Autodesk Inventor part; units mm, degrees
ref_plane "YZ Plane" through (0, 0, 0) normal (1, 0, 0) x (0, 1, 0)
ref_plane "XZ Plane" through (0, 0, 0) normal (0, 1, 0) x (-1, 0, 0)
ref_plane "XY Plane" through (0, 0, 0) normal (0, 0, 1) x (1, 0, 0)
sketch "Sketch1" plane through (0, 0, 0) normal (0, 1, 0) x (-1, 0, 0)
  line L0 (6.1765, 12) -> (-98.8235, 12)
  line L1 (-98.8235, 12) -> (-98.8235, -102)
  line L2 (-6.8235, 12) -> (-6.8235, 18)
  line L3 (-6.8235, 18) -> (6.1765, 18)
  line L4 (6.1765, 18) -> (6.1765, 12)
  line L5 (-98.8235, 12) -> (-98.8235, 18)
  line L6 (-98.8235, 18) -> (-85.8235, 18)
  line L7 (-85.8235, 18) -> (-85.8235, 12)
  line L8 (-98.8235, -102) -> (-85.8235, -87.8857)
  line L9 (-6.8235, -2.1143) -> (6.1765, 12)
  line L10 (-98.8235, -102) -> (-80.8235, -102)
  line L11 (6.1765, 12) -> (-80.8235, -102)
  point P0 (0, 0)
  point P1 (-96.8235, 18)
  point P2 (-96.8235, 18)
  dimension "d0" = 114
  dimension "d1" = 105
  dimension "d2" = 13
  dimension "d3" = 6
  dimension "d4" = 13
  dimension "d5" = 6
  dimension "d6" = 18
extrude "Extrusion1" add sketch "Sketch1" along normal blind 2
sketch "Sketch2" plane through (0, 2, 0) normal (0, 1, 0) x (1, 0, 0)
  line L0 (98.8235, 102) -> (80.8235, 102)
  line L1 (95.8235, 102) -> (87.8235, 102)
  line L2 (87.8235, 102) -> (87.8235, 82)
  line L3 (87.8235, 82) -> (95.8235, 82)
  line L4 (95.8235, 82) -> (95.8235, 102)
  line L5 (98.8235, -18) -> (98.8235, 102)
  point P0 (0, 0)
  dimension "d9" = 20
  dimension "d10" = 8
  dimension "d11" = 3
extrude "Extrusion2" add sketch "Sketch2" along normal blind 3
fillet "Fillet1" radius 4 2 edges at (87.8235, 5, -92) (95.8235, 5, -92)
sketch "Sketch3" plane through (0, 0, 0) normal (0, -1, 0) x (1, 0, 0)
  line L0 (87.8235, -102) -> (80.8235, -102)
  line L1 (87.8235, -102) -> (95.8235, -102)
  line L2 (95.8235, -102) -> (95.8235, -82)
  line L3 (95.8235, -82) -> (87.8235, -82)
  line L4 (87.8235, -82) -> (87.8235, -102)
  line L5 (98.8235, 18) -> (98.8235, -102)
  point P0 (0, 0)
  dimension "d16" = 20
  dimension "d17" = 8
  dimension "d18" = 3
extrude "Extrusion3" add sketch "Sketch3" along normal blind 3
fillet "Fillet3" radius 4 2 edges at (87.8235, -3, -92) (95.8235, -3, -92)
sketch "Sketch4" plane through (80.8235, 0, -102) normal (0, 0, -1) x (-1, 0, 0)
  arc A0 (-15, 0) -> (-11.127, -3) centre (-11.127, 1) ccw
  line L0 (-11.127, 4.8105) -> (-11.127, -3)
  circle A1 centre (-11.127, 1) radius 2.5
  point P0 (80.8235, 0)
  dimension "d25" = 5
extrude "Extrusion4" cut sketch "Sketch4" against normal blind 5
sketch "Sketch5" plane through (0, 2, 0) normal (0, 1, 0) x (1, 0, 0)
  line L0 (85.8235, -12) -> (85.8235, -18)
  line L1 (85.8235, -12) -> (98.8235, -12)
  line L2 (98.8235, -18) -> (98.8235, 102)
  circle A0 centre (92.3235, -12) radius 2.5
  point P0 (0, 0)
  dimension "d26" = 5
extrude "Extrusion5" cut sketch "Sketch5" against normal blind 2
sketch "Sketch6" plane through (0, 2, 0) normal (0, 1, 0) x (1, 0, 0)
  line L0 (-6.1765, -12) -> (-6.1765, -18)
  line L1 (6.8235, -18) -> (6.8235, -12)
  line L2 (-6.1765, -12) -> (6.8235, -12)
  circle A0 centre (0.3235, -12) radius 2.5
  point P0 (0, 0)
  dimension "d29" = 5
  dimension "d32" = 6.5
  dimension "d33" = 6
extrude "Extrusion6" cut sketch "Sketch6" against normal blind 2
equation "\"d23\" = d22"
properties part number "Triangle"
Can you work these out from the model? Positions are in its coordinate system, mm. A direction names the side the tool comes from. Give positions to 0.01 mm unless a question says otherwise; leave off trailing zeros. Loops run counter-clockwise (first coordinate to the right, second up) from the corner with the lowest first, then second, coordinate; pieces in that order, holes last. Notation, with made-up numbers: (23, 52) -> (76, 52) arc R31 cw to (76, 90) -> close; hole circle Ø6 at (-29.75, 82). An arc over 180 degrees is marked (long way). Write item = value, one per line.
1) Suppose I cut it at B-B on x = 52. Write out the boundary of the cut face in (y, z).
Check result:
outline = (0, -64.23) -> (2, -64.23) -> (2, 12) -> (0, 12) -> close
2) Thinking about a two-plate mould opening in X: for faces 1 (the flat face through (92, 1, -97)), 2 (the cylindrical face through (94.43, 4.14, -91.86)), 3 (the flat face through (92, -1, -82)), which applies, released by +X, released by -X, zero draft, split by the parting line, or undercut?
Check result:
face_1 = undercut
face_2 = released by +X
face_3 = zero draft
3) Suppose I cut it at A-A on z = -89. Write out the boundary of the cut face in (x, y).
Check result:
outline = (70.9, 0) -> (87.82, 0) arc R4 ccw to (91.7, -3) -> (91.95, -3) arc R4 ccw to (95.82, 0) -> (98.82, 0) -> (98.82, 2) -> (95.82, 2) arc R4 ccw to (91.95, 5) -> (91.7, 5) arc R4 ccw to (87.82, 2) -> (70.9, 2) -> close
4) For faces 4 (the cylindrical face through (94.71, 1.01, 11.25)), 5 (the flat face through (92, 3, -82)), 6 (the cylindrical face through (89.566, 1.751, -99.535)), which set-ups out of +Z, -Z, +X, -X, +Y, -Y let a thin tool reach every point of the face, with its end or its side?
Check result:
face_4 = +Y, -Y
face_5 = +Z, +X, -X, +Y
face_6 = -Z
5) Suppose I cut it at C-C on x = 65. Write out the boundary of the cut face in (y, z), then the cut area to 3 significant figures.
Check result:
outline = (0, -81.27) -> (2, -81.27) -> (2, 12) -> (0, 12) -> close
area = 187 mm2
6) I need wall thicknesses on L1, parallel to Y at x = 91.5, z = -6.5; L2, parallel to Z at x = 82, y = 0.25; L3, parallel to X at y = 1, z = -90. Which ranges of each line are inside material? Lowest first, please. Write a range as from..to.
Check result:
L1 = 0..2
L2 = -102..12
L3 = 71.67..98.82
7) Will these pins go through, and if not, where does the flat tip stop? pin 1 (4 mm diameter, centred on x = 73.5, y = 0, fed in from +Z); pin 2 (10 mm diameter, centred on x = 34.5, z = -4.5, fed in from -Y); pin 3 (5 mm diameter, centred on x = 57, z = -61.5, fed in from +Y).
Check result:
pin_1 = 12
pin_2 = 0
pin_3 = 2
